Geometry: final body of the model. Coordinates: model frame, mm. Face numbers are marked on the shaded views. A direction names the side the tool comes from. Coordinates: 2 decimals unless noted, no trailing zeros. Order: outer loops, then holes, each group sorted by start corner. A loop starts at its lowest first (then second) coordinate and runs counter-clockwise, first axis right, second up. Notation, with made-up numbers: (5.5, 50.5) - (57.5, 50.5) arc R12 cw to (57.5, 66.5) - close; hole circle Ø5 at (-34, 55.25). An arc over 180 degrees is marked (long way). Use a Markdown table: item, result. Add a question column.
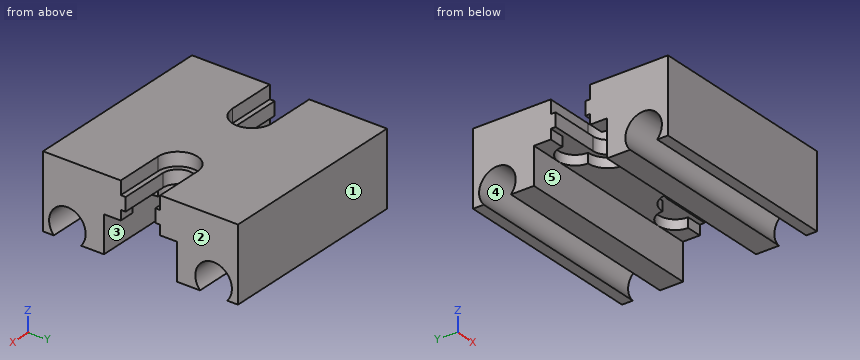
Autodesk Inventor part; units mm, degrees
ref_plane "YZ Plane" through (0, 0, 0) normal (1, 0, 0) x (0, 1, 0)
ref_plane "XZ Plane" through (0, 0, 0) normal (0, 1, 0) x (-1, 0, 0)
ref_plane "XY Plane" through (0, 0, 0) normal (0, 0, 1) x (1, 0, 0)
sketch "Sketch1" plane through (0, 0, 0) normal (0, 0, 1) x (1, 0, 0)
  line L0 (0, 0) -> (80, 0)
  line L1 (80, 0) -> (80, -80)
  line L2 (80, -80) -> (0, -80)
  line L3 (0, -80) -> (0, 0)
  dimension "d0" = 80
  dimension "d1" = 80
extrude "Extrusion1" add sketch "Sketch1" along normal blind 15
sketch "Sketch2" plane through (0, 0, 0) normal (0, 0, -1) x (-1, 0, 0)
  line L0 (0, 0) -> (-80, 0)
  circle A0 centre (-60, -40) radius 6.1
  line L1 (-80, 0) -> (-80, -80)
  line L2 (-60, -33.9) -> (-80, -33.9)
  line L3 (-80, -80) -> (-80, 0)
  line L4 (-60, -46.1) -> (-80, -46.1)
  line L5 (-80, -46.1) -> (-80, -33.9)
  dimension "d7" = 40
  dimension "d8" = 20
  dimension "d9" = 12.2
extrude "Extrusion2" cut sketch "Sketch2" against normal through all
sketch "Sketch3" plane through (0, 0, 0) normal (0, 0, -1) x (-1, 0, 0)
  arc A0 (-60, -46.1) -> (-60, -33.9) centre (-60, -40) ccw
  circle A1 centre (-60, -40) radius 8.1
  line L0 (-60, -31.9) -> (-80, -31.9)
  line L1 (-80, -33.9) -> (-80, 0)
  line L2 (-60, -48.1) -> (-80, -48.1)
  line L3 (-80, -48.1) -> (-80, -31.9)
  point P0 (0, 0)
  dimension "d12" = 16.2
extrude "Extrusion3" cut sketch "Sketch3" against normal blind 4
sketch "Sketch4" plane through (0, 0, 15) normal (0, 0, 1) x (1, 0, 0)
  line L0 (80, -31.9) -> (60, -31.9)
  arc A0 (60, -31.9) -> (60, -48.1) centre (60, -40) ccw
  line L1 (60, -48.1) -> (80, -48.1)
  line L2 (80, -46.1) -> (60, -46.1)
  arc A1 (60, -33.9) -> (60, -46.1) centre (60, -40) ccw
  line L3 (60, -33.9) -> (80, -33.9)
  line L4 (80, -33.9) -> (80, -31.9)
  line L5 (80, -33.9) -> (80, 0)
  line L6 (80, -46.1) -> (80, -48.1)
  line L7 (80, -80) -> (80, -46.1)
  point P0 (0, 0)
extrude "Extrusion4" cut sketch "Sketch4" against normal blind 5.5
sketch "Sketch5" plane through (0, 0, 0) normal (0, 0, -1) x (-1, 0, 0)
  arc A0 (-60, -46.1) -> (-60, -33.9) centre (-60, -40) ccw
  line L0 (-80, -31.9) -> (-60, -31.9)
  circle A1 centre (-60, -40) radius 8.1
  line L1 (-60, -31.9) -> (-60, -31.9)
  line L2 (-73.8, -31.9) -> (-73.8, -48.1)
  line L3 (-60, -48.1) -> (-60, -48.1)
  arc A2 (-60, -48.1) -> (-60, -31.9) centre (-60, -40) ccw
  line L4 (-60, -31.9) -> (-60, -31.9)
  line L5 (-60, -31.9) -> (-60, -31.9)
  line L6 (-60, -33.9) -> (-60, -46.1)
  arc A3 (-60, -31.9) -> (-73.8, -31.9) centre (-66.9, -31.9) ccw
  arc A4 (-73.8, -48.1) -> (-60, -48.1) centre (-66.9, -48.1) ccw
  point P0 (0, 0)
  dimension "d17" = 13.8
  dimension "d20" = 16.2
  dimension "d21" = 8.1
  dimension "d37" = 0
extrude "Extrusion5" cut sketch "Sketch5" against normal blind 4 contours A3 L0 | L0 A1 A4 L2
sketch "Sketch6" plane through (80, 0, 15) normal (1, 0, 0) x (0, 0, -1)
  line L0 (15, 0) -> (0, 0)
  line L1 (15, 0) -> (30, 0)
  line L2 (30, -25) -> (15, -25)
  line L3 (15, -25) -> (15, 0)
  line L4 (15, -80) -> (0, -80)
  line L5 (15, -80) -> (30, -80)
  line L6 (30, -55) -> (15, -55)
  line L7 (15, -55) -> (15, -80)
  arc A0 (30, -4.4098) -> (30, -15.5902) centre (25, -10) ccw
  arc A1 (30, -64.4098) -> (30, -75.5902) centre (25, -70) ccw
  line L8 (30, 0) -> (30, -4.4098)
  line L9 (30, -15.5902) -> (30, -25)
  line L10 (30, -80) -> (30, -75.5902)
  line L11 (30, -64.4098) -> (30, -55)
  dimension "d22" = 25
  dimension "d23" = 25
  dimension "d24" = 15
  dimension "d25" = 15
  dimension "d29" = 15
  dimension "d32" = 15
  dimension "d33" = 5
  dimension "d34" = 5
  dimension "d38" = 15
  dimension "d39" = 15
  dimension "d40" = 60
  dimension "d41" = 10
  dimension "d42" = 10
extrude "Extrusion6" add sketch "Sketch6" against normal blind 80
ref_plane "Work Plane1" through (40, -33.9, 4) normal (1, 0, 0) x (0, 0, -1)
mirror "Mirror1" about plane through (40, -33.9, 4) normal (1, 0, 0) of "Extrusion5", "Extrusion4", "Extrusion3", "Extrusion2"
equation "\"d24\" = d25"
equation "\"d32\" = d29"
equation "\"d34\" = d33"
equation "\"RodDiameter\" = 8"
equation "\"VerticalBearingOD\" = 16"
equation "\"PrintingClearance\" = 0.2"
equation "\"d31\" = d30"
properties part number "HotendMountCarriage"
1) Draft query along Y for the marked faces 1, 2 and 3. Return one class per face: released by +Y, released by -Y, zero draft, split by the parting line, or undercut.
2) Section query B-B (z = 3). Return the cut outline in (x, y), and give its area (3 significant figures).
3) Section query D-D (y = -40). Return the cut outline in (x, z), and give its area (3 significant figures).
4) First-contact query: pin 1 (24 mm diameter, centred on x = 50, y = -39, fed in from -Z). Flat tip, straight axial feed; report the tip coordinate or a pass-through.
5) Line query: line 1 (Y direction, x = 60, z = -10); line 2 (Y direction, x = 17, z = -7.25); line 3 (X direction, y = -52.5, z = 2.5). Output: solid intervals per line, ascending. Write a range as from..to.
6) Section query C-C (x = 69.5). Return the cut outline in (y, z), and give its area (3 significant figures).
7) Section query A-A (z = -10). Return the cut outline in (x, y).
8) Access query for the marked faces 4 and 5. Directions: +Z, -Z, +X, -X, +Y, -Y. A direction counts if a zero-diameter tool reaches every point of the face in a straight line with its end or side. Return the directions, or none.
From the geometry:
| question | item | result |
|---|---|---|
| 1 | face 1 | released by +Y |
| 1 | face 2 | zero draft |
| 1 | face 3 | undercut |
| 2 | outline | (0, -80) - (80, -80) - (80, -48.1) - (73.8, -48.1) arc R6.9 cw to (60, -48.1) arc R8.1 cw to (60, -31.9) arc R6.9 cw to (73.8, -31.9) - (80, -31.9) - (80, 0) - (0, 0) - (0, -31.9) - (6.2, -31.9) arc R6.9 cw to (20, -31.9) arc R8.1 cw to (20, -48.1) arc R6.9 cw to (6.2, -48.1) - (0, -48.1) - close |
| 2 | area | 5,250 mm^2 |
| 3 | outline | (26.1, 4) - (28.1, 4) - (28.1, 0) - (51.9, 0) - (51.9, 4) - (53.9, 4) - (53.9, 9.5) - (51.9, 9.5) - (51.9, 15) - (28.1, 15) - (28.1, 9.5) - (26.1, 9.5) - close |
| 3 | area | 379 mm^2 |
| 4 | pin 1 | stops at z = 0 |
| 5 | line 1 | y = -80..-77.5, -62.5..-55, -25..-17.5, -2.5..0 |
| 5 | line 2 | y = -80..-76.98, -63.02..-55, -25..-16.98, -3.02..0 |
| 5 | line 3 | x = 0..7.78, 18.42..61.58, 72.22..80 |
| 6 | outline | (-80, -15) - (-75.59, -15) arc R7.5 cw (long way) to (-64.41, -15) - (-55, -15) - (-55, 0) - (-54.49, 0) - (-54.49, 4) - (-46.1, 4) - (-46.1, 9.5) - (-48.1, 9.5) - (-48.1, 15) - (-80, 15) - close; (-33.9, 4) - (-25.51, 4) - (-25.51, 0) - (-25, 0) - (-25, -15) - (-15.59, -15) arc R7.5 cw (long way) to (-4.41, -15) - (0, -15) - (0, 15) - (-31.9, 15) - (-31.9, 9.5) - (-33.9, 9.5) - close |
| 6 | area | 1,360 mm^2 |
| 7 | outline | (0, -80) - (80, -80) - (80, -77.5) - (0, -77.5) - close; (0, -62.5) - (80, -62.5) - (80, -55) - (0, -55) - close; (0, -25) - (80, -25) - (80, -17.5) - (0, -17.5) - close; (0, -2.5) - (80, -2.5) - (80, 0) - (0, 0) - close |
| 8 | face 4 | +X, -X |
| 8 | face 5 | -Z, +X, -X |
